Check sheet for the drawn part. Datum: minimum x, y, z corner. Units: mm. Round coordinates to 2 decimals unless told otherwise and drop trailing zeros. Order: outer loops, then holes, each group sorted by start corner. A loop starts at its lowest first (then second) coordinate and runs counter-clockwise, first axis right, second up. Notation, with made-up numbers: M 28,5 L 83,5 A25 cw 83,24 Z; hole C 24.25,64.5 d10. An arc over 180 degrees is marked long. Answer as a JSON object with one key per item and string values. Group by question number.
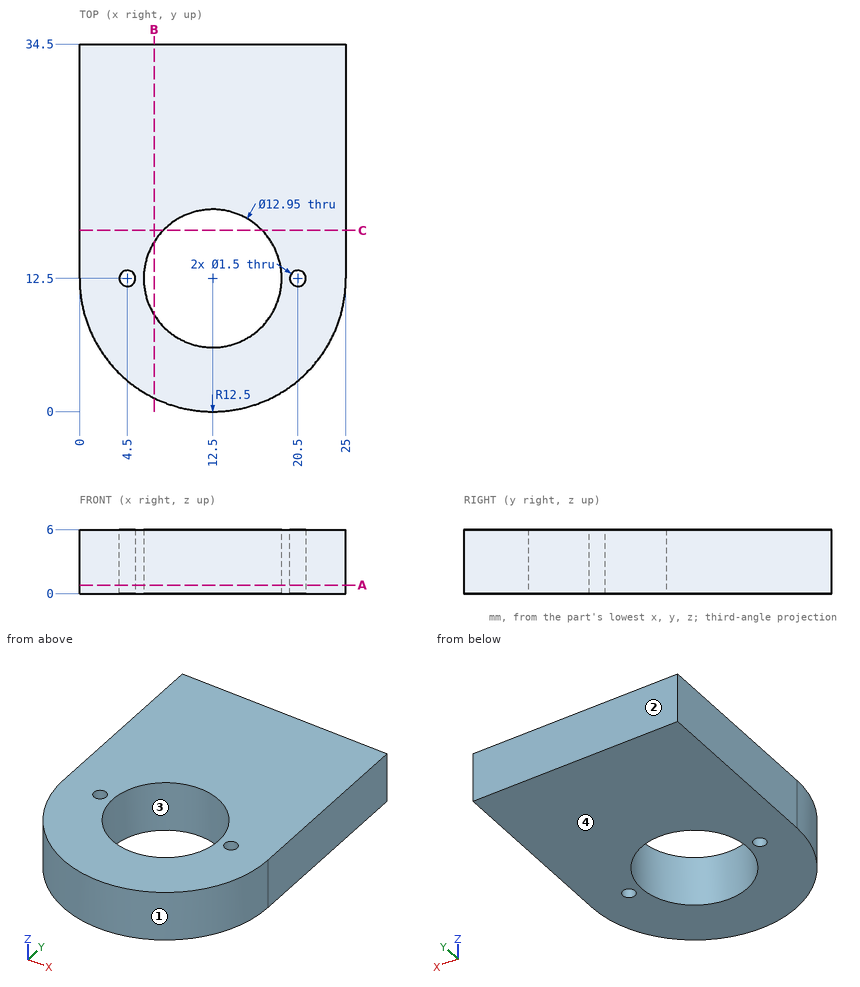
1) Sectioned sample at A-A (z = 0.8). Record the boundary of the cut face in (x, y) (3 decimals).
2) Thickness scan on line 1 along Y through (x, z) = (9, 1.25); line 2 along X through (y, z) = (18.5, 1.05); line 3 along X through (y, z) = (11, 2.2). Record the ranges inside material, lowest first. Write a range as [from, to].
3) Sectioned sample at B-B (x = 7). Record the boundary of the cut face in (y, z), then the cut area to 3 significant figures.
4) Go/stop test with flat-tipped pins: P1, Ø8, axis at x = 12.5, y = 12.5, coming from the -Z side; P2, Ø1, axis at y = 30.5, z = 3.5, coming from the -X side. Record where each tip stops, or that it passes through.
5) Sectioned sample at C-C (y = 17). Record the boundary of the cut face in (x, z).
6) Release check for a two-part mould opening along Y. For the marked faces 1, 2, 3 and 4 record: +Y half, -Y half, draft (parallel to the pull), parting line (faces both ways), or undercut.
Final values:
{
 "1": {"outline": "M 0,12.5 A12.5 ccw 25,12.5 L 25,34.5 L 0,34.5 Z; hole C 4.5,12.5 d1.5; hole C 12.5,12.5 d12.95; hole C 20.5,12.5 d1.5"},
 "2": {"line 1": "y = [0.5, 7.05], [17.95, 34.5]", "line 2": "x = [0, 10.07], [14.93, 25]", "line 3": "x = [0.09, 6.2], [18.8, 24.91]"},
 "3": {"outline": "M 1.28,0 L 9.08,0 L 9.08,6 L 1.28,6 Z; M 15.92,0 L 34.5,0 L 34.5,6 L 15.92,6 Z", "area": "158 mm^2"},
 "4": {"P1": "passes through", "P2": "stops at x = 0"},
 "5": {"outline": "M 0,0 L 7.84,0 L 7.84,6 L 0,6 Z; M 17.16,0 L 25,0 L 25,6 L 17.16,6 Z"},
 "6": {"face 1": "-Y half", "face 2": "+Y half", "face 3": "undercut", "face 4": "draft"}
}
